Model file for the job. Use its own axes, mm. Face numbers are marked on the shaded views. Coordinates: 2 decimals unless noted, no trailing zeros. Order: outer loops, then holes, each group sorted by start corner. A loop starts at its lowest first (then second) coordinate and runs counter-clockwise, first axis right, second up. Notation, with made-up numbers: (63, 0) -> (115, 0) arc R26 cw to (115, 16) -> close; hole circle Ø2 at (51.25, -36). An arc over 180 degrees is marked (long way). Write item = value, one per line. Start each with the question number.
Q1. Mould opens along Y. For the marked faces 1, 2 and 3 say: +Y half, -Y half, draft (parallel to the pull), parting line (faces both ways), or undercut.
Q2. Cut at B-B, the plane z = 15. List the corners of the cut face in (x, y).
Q3. Cut at A-A, the plane x = 0. List the corners of the cut face in (y, z), plus the area to 3 significant figures.
Q4. Flat gauge pins, fed straight in: pin 1 (5 mm diameter, centred on x = -18, z = 15.5, fed in from +Y); pin 2 (1 mm diameter, centred on x = 28.5, z = 10.5, fed in from +Y); pin 3 (2.5 mm diameter, centred on x = 0, y = 23.5, fed in from +Z); pin 4 (1 mm diameter, centred on x = -13, z = 5.5, fed in from -Y). Where does each tip first touch, or does it go through?
Q5. Cut at D-D, the plane z = 7.5. List the corners of the cut face in (x, y).
Q6. Cut at C-C, the plane y = 0. List the corners of the cut face in (x, z), plus the area to 3 significant figures.
Q7. Wall check: line 1 (Y direction, x = 21, z = 22); line 2 (Z direction, x = 11, y = 15); line 3 (X direction, y = -20, z = 10.5). Give the ranges that are in metal, low to high. Write a range as from..to.
from build123d import *

# Parameters (mm, degrees)
CROQUIS1_R              = 30
SALIENTE_EXTRUIR1_DEPTH = 30
VACIADO1_T              = -2
REDONDEO1_R             = 2
CORTAR_EXTRUIR1_REACH   = 75.485
CROQUIS3_R              = 10.1
CORTAR_EXTRUIR2_REACH   = 53.962
CROQUIS5_R              = 1.4
CHAFL_N1_SIZE           = 1.6
CROQUIS11_R             = 1.25
CROQUIS11_W             = 12
CROQUIS11_H             = 8
CORTAR_EXTRUIR3_DEPTH   = 52.961524343


with BuildPart() as part:
    # Croquis1 → Saliente-Extruir1 (new body)
    with BuildSketch(Plane.XY):
        Circle(CROQUIS1_R)
    extrude(amount=SALIENTE_EXTRUIR1_DEPTH)

    # Vaciado1
    vaciado1_openings = [part.faces().sort_by_distance(p)[0] for p in [
        (0, 0, 0),
    ]]
    offset(amount=VACIADO1_T, openings=vaciado1_openings, kind=Kind.INTERSECTION)

    # Redondeo1
    redondeo1_edges = [part.edges().sort_by_distance(p)[0] for p in [
        (-30, 0, 30),
        (-28, 0, 28),
    ]]
    fillet(redondeo1_edges, radius=REDONDEO1_R)

    # Croquis3 → Cortar-Extruir1 (cut, up to next)
    with BuildSketch(Plane(origin=(30, 0, 30), x_dir=(0, 0, -1), z_dir=(1, 0, 0)), mode=Mode.PRIVATE) as cortar_extruir1_sk1:
        with Locations((15, -7.5)):
            Circle(CROQUIS3_R)
    cortar_extruir1_tool1 = extrude(cortar_extruir1_sk1.sketch, amount=-CORTAR_EXTRUIR1_REACH, mode=Mode.PRIVATE) & part.part
    add(cortar_extruir1_tool1.solids().sort_by_distance((30, -7.5, 15))[0], mode=Mode.SUBTRACT)

    # Croquis5 → Cortar-Extruir2 (cut, up to next)
    with BuildSketch(Plane.XY.offset(30), mode=Mode.PRIVATE) as cortar_extruir2_sk1:
        with Locations((0, 23.5)):
            Circle(CROQUIS5_R)
    cortar_extruir2_tool1 = extrude(cortar_extruir2_sk1.sketch, amount=-CORTAR_EXTRUIR2_REACH, mode=Mode.PRIVATE) & part.part
    # Croquis5 → Cortar-Extruir2 (cut, up to next)
    with BuildSketch(Plane.XY.offset(30), mode=Mode.PRIVATE) as cortar_extruir2_sk2:
        with Locations((-22, 0)):
            Circle(CROQUIS5_R)
    cortar_extruir2_tool2 = extrude(cortar_extruir2_sk2.sketch, amount=-CORTAR_EXTRUIR2_REACH, mode=Mode.PRIVATE) & part.part
    # Croquis5 → Cortar-Extruir2 (cut, up to next)
    with BuildSketch(Plane.XY.offset(30), mode=Mode.PRIVATE) as cortar_extruir2_sk3:
        with Locations((0, -23.5)):
            Circle(CROQUIS5_R)
    cortar_extruir2_tool3 = extrude(cortar_extruir2_sk3.sketch, amount=-CORTAR_EXTRUIR2_REACH, mode=Mode.PRIVATE) & part.part
    add(cortar_extruir2_tool1.solids().sort_by_distance((0, 23.5, 30))[0], mode=Mode.SUBTRACT)
    add(cortar_extruir2_tool2.solids().sort_by_distance((-22, 0, 30))[0], mode=Mode.SUBTRACT)
    add(cortar_extruir2_tool3.solids().sort_by_distance((0, -23.5, 30))[0], mode=Mode.SUBTRACT)

    # Chaflán1
    chafl_n1_edges = [part.edges().sort_by_distance(p)[0] for p in [
        (-1.4, 23.5, 30),
        (-23.4, 0, 30),
        (-1.4, -23.5, 30),
    ]]
    chamfer(chafl_n1_edges, length=CHAFL_N1_SIZE)

    # Croquis11 → Cortar-Extruir3 (cut, through all)
    with BuildSketch(Plane(origin=(0, 0, 0), x_dir=(0, 0, -1), z_dir=(1, 0, 0))):
        with Locations(Location((-22.5, 19.842217067, 0), (0, 0, 180))):
            Circle(CROQUIS11_R)
        with Locations(Location((-7.5, 19.842217067, 0), (0, 0, 180))):
            Circle(CROQUIS11_R)
        with Locations((-9.85, 11.842217067)):
            Rectangle(CROQUIS11_W, CROQUIS11_H)
    extrude(amount=CORTAR_EXTRUIR3_DEPTH, mode=Mode.SUBTRACT)


solid = part.part
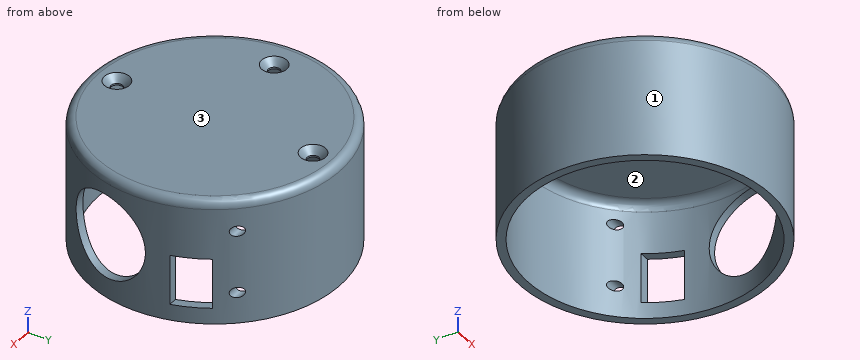
Here are the results:
q1.face_1 = parting line
q1.face_2 = undercut
q1.face_3 = draft
q2.outline = (21.78, -17.6) arc R28 cw (long way) to (23.09, 15.84) -> (25.48, 15.84) arc R30 ccw (long way) to (24.29, -17.6) -> close; (26.88, 7.84) arc R28 cw to (27.88, 2.6) -> (29.89, 2.6) arc R30 ccw to (28.96, 7.84) -> close
q3.outline = (-30, 0) -> (-28, 0) -> (-28, 26) arc R2 cw to (-26, 28) -> (-24.9, 28) -> (-24.9, 28.4) -> (-26.5, 30) -> (-28, 30) arc R2 ccw to (-30, 28) -> close; (-22.1, 28) -> (22.1, 28) -> (22.1, 28.4) -> (20.5, 30) -> (-20.5, 30) -> (-22.1, 28.4) -> close; (24.9, 28) -> (26, 28) arc R2 cw to (28, 26) -> (28, 0) -> (30, 0) -> (30, 28) arc R2 ccw to (28, 30) -> (26.5, 30) -> (24.9, 28.4) -> close
q3.area = 216 mm²
q4.pin_1 = 25.69
q4.pin_2 = 7.84
q4.pin_3 = through
q4.pin_4 = -27.27
q5.outline = (18.42, 21.09) -> (21.33, 21.09) arc R30 ccw (long way) to (26.39, -14.26) -> (24.09, -14.26) arc R28 cw (long way) to start; (20.94, 18.59) arc R28 cw to (23.09, 15.84) -> (25.48, 15.84) arc R30 ccw to (23.54, 18.59) -> close; (26.88, 7.84) arc R28 cw to (27.99, -0.74) -> (29.99, -0.74) arc R30 ccw to (28.96, 7.84) -> close
q6.outline = (-30, 0) -> (-28, 0) -> (-28, 26) arc R2 cw to (-26, 28) -> (-23.4, 28) -> (-23.4, 28.4) -> (-25, 30) -> (-28, 30) arc R2 ccw to (-30, 28) -> close; (-20.6, 28) -> (26, 28) arc R2 cw to (28, 26) -> (28, 21.76) -> (30, 21.76) -> (30, 28) arc R2 ccw to (28, 30) -> (-19, 30) -> (-20.6, 28.4) -> close; (28, 0) -> (30, 0) -> (30, 8.24) -> (28, 8.24) -> close
q6.area = 197 mm²
q7.line_1 = -21.42..-18.52, 18.52..18.7, 20.99..21.42
q7.line_2 = 28..30
q7.line_3 = -22.36..-19.6, 19.6..22.36
